from build123d import *

# Parameters (mm, degrees)
SKETCH1_W           = 157.48
SKETCH1_H           = 106.68
BOSS_EXTRUDE1_DEPTH = 2.54
SKETCH2_W           = 152.654
SKETCH2_H           = 101.854
BOSS_EXTRUDE2_DEPTH = 5.08
SKETCH3_W           = 149.606
SKETCH3_H           = 98.806
CUT_EXTRUDE1_DEPTH  = 2.54
SKETCH4_W           = 99.568
SKETCH4_H           = 58.42
CUT_EXTRUDE2_DEPTH  = 96.241532957


with BuildPart() as part:
    # Sketch1 → Boss-Extrude1 (new body)
    with BuildSketch(Plane.XY):
        Rectangle(SKETCH1_W, SKETCH1_H)
    extrude(amount=BOSS_EXTRUDE1_DEPTH)

    # Sketch2 → Boss-Extrude2 (add)
    with BuildSketch(Plane.XY.offset(2.54)):
        Rectangle(SKETCH2_W, SKETCH2_H)
    extrude(amount=BOSS_EXTRUDE2_DEPTH)

    # Sketch3 → Cut-Extrude1 (cut)
    with BuildSketch(Plane.XY.offset(7.62)):
        Rectangle(SKETCH3_W, SKETCH3_H)
    extrude(amount=-CUT_EXTRUDE1_DEPTH, mode=Mode.SUBTRACT)

    # Sketch4 → Cut-Extrude2 (cut, through all)
    with BuildSketch(Plane.XY.offset(5.08)):
        Rectangle(SKETCH4_W, SKETCH4_H)
    extrude(amount=-CUT_EXTRUDE2_DEPTH, mode=Mode.SUBTRACT)


solid = part.part
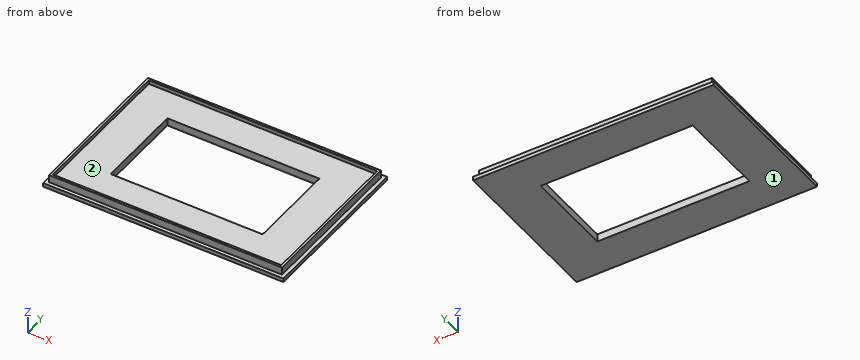
Source: CAD feature listing. Evaluate the final solid. Frame: model axes, mm. Face numbers are marked on the shaded views. Give positions to 0.01 mm unless a question says otherwise; leave off trailing zeros. Write each loop counter-clockwise with the first axis right and the second up, starting at its lowest first coordinate (ties: lowest second). Pieces come first, ordered by that corner, then holes. Notation, with made-up numbers: (44, -7.5) - (97, -7.5) arc R25 cw to (97, 21.5) - close; hole circle Ø11 at (19.25, 79.25). An arc over 180 degrees is marked (long way). Write item = value, one per line. Start each with the question number.
Q1. Cut plane D-D, the plane y = -43. Return loops of the section in (x, z), then the cut area to 3 significant figures.
Q2. Cut plane B-B, the plane x = 27. Return loops of the section in (y, z), then the cut area to 3 significant figures.
Q3. Draft query along X for the marked faces 1 and 2. Return one class per face: +X half, -X half, draft (parallel to the pull), parting line (faces both ways), or undercut.
Q4. Pin query (flat end, axial travel): pin 1 Ø12 at (x, y) = (-19.5, -40.5) entering from +Z; pin 2 Ø2 at (x, z) = (-19.5, 6.5) entering from +Y; pin 3 Ø2.5 at (x, z) = (12.5, 5) entering from -Y. Return the tip coordinate at first contact, or that it passes through.
Q5. Cut plane C-C, the plane z = 1.25. Return loops of the section in (x, y).
Q6. Material intervals for probe 1 along Y at (x, z) = (4, 3.5); probe 2 along X at (y, z) = (-12.5, 0.5); probe 3 along Y at (x, z) = (67, 7.25), sorted ascending.
Q7. Cut plane A-A, the plane y = -18. Return loops of the section in (x, z), then the cut area to 3 significant figures.
Computed values:
q1.outline = (-78.74, 0) - (78.74, 0) - (78.74, 2.54) - (76.33, 2.54) - (76.33, 7.62) - (74.8, 7.62) - (74.8, 5.08) - (-74.8, 5.08) - (-74.8, 7.62) - (-76.33, 7.62) - (-76.33, 2.54) - (-78.74, 2.54) - close
q1.area = 795 mm²
q2.outline = (-53.34, 0) - (-29.21, 0) - (-29.21, 5.08) - (-49.4, 5.08) - (-49.4, 7.62) - (-50.93, 7.62) - (-50.93, 2.54) - (-53.34, 2.54) - close; (29.21, 0) - (53.34, 0) - (53.34, 2.54) - (50.93, 2.54) - (50.93, 7.62) - (49.4, 7.62) - (49.4, 5.08) - (29.21, 5.08) - close
q2.area = 241 mm²
q3.face_1 = draft
q3.face_2 = undercut
q4.pin_1 = 5.08
q4.pin_2 = 50.93
q4.pin_3 = -50.93
q5.outline = (-78.74, -53.34) - (78.74, -53.34) - (78.74, 53.34) - (-78.74, 53.34) - close; hole (-49.78, -29.21) - (49.78, -29.21) - (49.78, 29.21) - (-49.78, 29.21) - close
q6.probe_1 = -50.93 to -29.21, 29.21 to 50.93
q6.probe_2 = -78.74 to -49.78, 49.78 to 78.74
q6.probe_3 = -50.93 to -49.4, 49.4 to 50.93
q7.outline = (-78.74, 0) - (-49.78, 0) - (-49.78, 5.08) - (-74.8, 5.08) - (-74.8, 7.62) - (-76.33, 7.62) - (-76.33, 2.54) - (-78.74, 2.54) - close; (49.78, 0) - (78.74, 0) - (78.74, 2.54) - (76.33, 2.54) - (76.33, 7.62) - (74.8, 7.62) - (74.8, 5.08) - (49.78, 5.08) - close
q7.area = 290 mm²
